```python
from build123d import *

# Parameters (mm, degrees)
EXTRUDE_1_DEPTH     = 5
SKETCH_7_R          = 20
EXTRUDE_3_DEPTH     = 10
CUT_EXTRUDE_2_REACH = 89.892
SKETCH_8_R          = 1.65
CUT_EXTRUDE_3_REACH = 89.464
SKETCH_9_R          = 2.1


with BuildPart() as part:
    # 草图1 → 凸台-拉伸1 (new body)
    with BuildSketch(Plane(origin=(0, 0, 0), x_dir=(1, 0, 0), z_dir=(0, 1, 0))):
        with BuildLine():
            Line((-65, 12.5), (65, 12.5))
            ThreePointArc((65, 12.5), (77.5, 0), (65, -12.5))
            Line((65, -12.5), (-65, -12.5))
            ThreePointArc((-65, -12.5), (-77.5, 0), (-65, 12.5))
        make_face()
    extrude(amount=EXTRUDE_1_DEPTH)

    # 草图7 → 凸台-拉伸3 (add)
    with BuildSketch(Plane(origin=(0, 0, 0), x_dir=(1, 0, 0), z_dir=(0, 1, 0))):
        with Locations(Location((65, 0, 0), (0, 0, 141.317812547))):
            Circle(SKETCH_7_R)
    extrude(amount=EXTRUDE_3_DEPTH)

    # 草图8 → 切除-拉伸2 (cut, up to next)
    with BuildSketch(Plane(origin=(0, 10, 0), x_dir=(1, 0, 0), z_dir=(0, 1, 0)), mode=Mode.PRIVATE) as cut_extrude_2_sk1:
        with Locations(Location((56.161165235, 8.838834765, 0), (0, 0, 270))):
            Circle(SKETCH_8_R)
    cut_extrude_2_tool1 = extrude(cut_extrude_2_sk1.sketch, amount=-CUT_EXTRUDE_2_REACH, mode=Mode.PRIVATE) & part.part
    # 草图8 → 切除-拉伸2 (cut, up to next)
    with BuildSketch(Plane(origin=(0, 10, 0), x_dir=(1, 0, 0), z_dir=(0, 1, 0)), mode=Mode.PRIVATE) as cut_extrude_2_sk2:
        with Locations(Location((73.838834765, 8.838834765, 0), (0, 0, 270))):
            Circle(SKETCH_8_R)
    cut_extrude_2_tool2 = extrude(cut_extrude_2_sk2.sketch, amount=-CUT_EXTRUDE_2_REACH, mode=Mode.PRIVATE) & part.part
    # 草图8 → 切除-拉伸2 (cut, up to next)
    with BuildSketch(Plane(origin=(0, 10, 0), x_dir=(1, 0, 0), z_dir=(0, 1, 0)), mode=Mode.PRIVATE) as cut_extrude_2_sk3:
        with Locations(Location((73.838834765, -8.838834765, 0), (0, 0, 270))):
            Circle(SKETCH_8_R)
    cut_extrude_2_tool3 = extrude(cut_extrude_2_sk3.sketch, amount=-CUT_EXTRUDE_2_REACH, mode=Mode.PRIVATE) & part.part
    # 草图8 → 切除-拉伸2 (cut, up to next)
    with BuildSketch(Plane(origin=(0, 10, 0), x_dir=(1, 0, 0), z_dir=(0, 1, 0)), mode=Mode.PRIVATE) as cut_extrude_2_sk4:
        with Locations(Location((56.161165235, -8.838834765, 0), (0, 0, 270))):
            Circle(SKETCH_8_R)
    cut_extrude_2_tool4 = extrude(cut_extrude_2_sk4.sketch, amount=-CUT_EXTRUDE_2_REACH, mode=Mode.PRIVATE) & part.part
    add(cut_extrude_2_tool1.solids().sort_by_distance((56.161165, 10, -8.838835))[0], mode=Mode.SUBTRACT)
    add(cut_extrude_2_tool2.solids().sort_by_distance((73.838835, 10, -8.838835))[0], mode=Mode.SUBTRACT)
    add(cut_extrude_2_tool3.solids().sort_by_distance((73.838835, 10, 8.838835))[0], mode=Mode.SUBTRACT)
    add(cut_extrude_2_tool4.solids().sort_by_distance((56.161165, 10, 8.838835))[0], mode=Mode.SUBTRACT)

    # 草图9 → 切除-拉伸3 (cut, up to next)
    with BuildSketch(Plane(origin=(0, 5, 0), x_dir=(1, 0, 0), z_dir=(0, 1, 0)), mode=Mode.PRIVATE) as cut_extrude_3_sk1:
        with Locations(Location((-65, 0, 0), (0, 0, 270))):
            Circle(SKETCH_9_R)
    cut_extrude_3_tool1 = extrude(cut_extrude_3_sk1.sketch, amount=-CUT_EXTRUDE_3_REACH, mode=Mode.PRIVATE) & part.part
    add(cut_extrude_3_tool1.solids().sort_by_distance((-65, 5, 0))[0], mode=Mode.SUBTRACT)


solid = part.part
```
Geometry check sheet. Reference: the model listing, model coordinates, mm. A direction names the side the tool comes from. Round coordinates to 2 decimals unless told otherwise and drop trailing zeros. Loops run counter-clockwise (first coordinate to the right, second up) from the corner with the lowest first, then second, coordinate; pieces in that order, holes last. Notation, with made-up numbers: (36.25, 83) - (40.25, 83) arc R14 ccw to (40.25, 97) - close; hole circle Ø3 at (60, -12.5). An arc over 180 degrees is marked (long way). Use a Markdown table: item, result.
Q1. Material ranges on line 1 (Z direction, x = 56, y = 7.75); line 2 (Z direction, x = -46.5, y = 3.25); line 3 (Y direction, x = 28, z = -11.5), recorded low to high.
Solutions:
| item | result |
|---|---|
| line 1 | z = -17.86 to -10.48, -7.2 to 7.2, 10.48 to 17.86 |
| line 2 | z = -12.5 to 12.5 |
| line 3 | y = 0 to 5 |
Q2. Cross-section at C-C on x = -36. Record the cut outline in (y, z).
Solutions:
| item | result |
|---|---|
| outline | (0, -12.5) - (5, -12.5) - (5, 12.5) - (0, 12.5) - close |
Q3. Cross-section at D-D on z = 16. Record the cut outline in (x, y), plus the area to 3 significant figures.
Solutions:
| item | result |
|---|---|
| outline | (53, 0) - (77, 0) - (77, 10) - (53, 10) - close |
| area | 240 mm2 |
Q4. Cross-section at A-A on z = 0. Record the cut outline in (x, y).
Solutions:
| item | result |
|---|---|
| outline | (-77.5, 0) - (-67.1, 0) - (-67.1, 5) - (-77.5, 5) - close; (-62.9, 0) - (85, 0) - (85, 10) - (45, 10) - (45, 5) - (-62.9, 5) - close |
Q5. Draft check along Z on faces 1 (the cylindrical face through (73.911, 5.07, -10.487)), 2 (the flat face through (-13, 5, 0)), 3 (the flat face through (-7, 2, 12.5)), 4 (the cylindrical face through (-77.497, 2.465, 0.275)). Enter one of: released by +Z, released by -Z, zero draft, split by the parting line, or undercut.
Solutions:
| item | result |
|---|---|
| face 1 | undercut |
| face 2 | zero draft |
| face 3 | released by +Z |
| face 4 | split by the parting line |
Q6. Access from +Z, -Z, +X, -X, +Y, -Y to the whole of each face (thin tool, end or side, straight path). Record for faces 5 (the flat face through (-9, 2, -12.5)), 6 (the cylindrical face through (57.797, 5.07, -9.054)).
Solutions:
| item | result |
|---|---|
| face 5 | -Z, -X, +Y, -Y |
| face 6 | +Y, -Y |
Q7. Go/stop test with flat-tipped pins: P1, Ø2, axis at y = 8.5, z = -4, coming from the +X side; P2, Ø1.5, axis at x = 20, y = 3.5, coming from the +Z side; P3, Ø5.5, axis at x = -65, z = 0, coming from the +Y side. Record where each tip stops, or that it passes through.
Solutions:
| item | result |
|---|---|
| P1 | stops at x = 84.77 |
| P2 | stops at z = 12.5 |
| P3 | stops at y = 5 |
Q8. Cross-section at B-B on y = 7.25. Record the cut outline in (x, z), plus the area to 3 significant figures.
Solutions:
| item | result |
|---|---|
| outline | circle Ø40 at (65, 0); hole circle Ø3.3 at (56.16, -8.84); hole circle Ø3.3 at (56.16, 8.84); hole circle Ø3.3 at (73.84, -8.84); hole circle Ø3.3 at (73.84, 8.84) |
| area | 1,220 mm2 |
